The listing builds one solid part. Answer for the finished solid, in the listing's coordinates (mm). A direction names the side the tool comes from. Round coordinates to 2 decimals unless told otherwise and drop trailing zeros. Order: outer loops, then holes, each group sorted by start corner. A loop starts at its lowest first (then second) coordinate and runs counter-clockwise, first axis right, second up. Notation, with made-up numbers: (-25.75, 51) - (19.25, 51) arc R9 ccw to (19.25, 59) - close; hole circle Ø11 at (41.25, -33). An arc over 180 degrees is marked (long way). Use CSV: the item, a comma, the result in double quotes. Start each with the question number.
Item 1: Find section A-A, the plane x = 0. Give the vertices of the cut face in (y, z), plus the area to 3 significant figures.
Item 2: Find section B-B, the plane z = 0. Give the vertices of the cut face in (x, y).
Item 3: Find section C-C, the plane x = 14. Give the vertices of the cut face in (y, z).
Item 4: Determine the mould class of faces 1 (the cylindrical face through (-10.74, 15.19, -2.38)), 2 (the cylindrical face through (16.539, 6.134, 11.127)), 3 (the flat face through (-5, 7.3, -10)) for opening direction X: +X half, -X half, draft (parallel to the pull), parting line (faces both ways), or undercut.
Item 5: Straight lines are drawn through the part: line 1 along Y through (x, z) = (-6.5, 13.5); line 2 along Z through (x, y) = (-4, 13); line 3 along X through (y, z) = (13.75, 6.5). For each, find the intervals that lie inside material, in ascending order. Write a range as [from, to].
Item 6: Flat-ended cylindrical pins translate along their axes: P1, Ø6, axis at x = 14.71, z = 9.14, coming from the -Y side; P2, Ø1, axis at x = 17, z = 17, coming from the -Y side; P3, Ø5, axis at x = 8, z = 17.5, coming from the +Y side; P4, Ø2, axis at x = 6, y = 17, coming from the +Z side. Find the tip coordinate at first contact, or state that the pin passes through.
Item 7: For faces 4 (the cylindrical face through (-2.44, 11.49, 0.54)), 5 (the flat face through (-5, 5, -10)), determine the directions among +Z, -Z, +X, -X, +Y, -Y from which every point of the face is accessible in a straight line to the end or side of a thin tool.
Item 8: Find section D-D, the plane y = 21.25. Give the vertices of the cut face in (x, z), plus the area to 3 significant figures.
```python
from build123d import *

# Parameters (mm, degrees)
SKETCH1_R           = 11
BOSS_EXTRUDE1_DEPTH = 5
SKETCH2_R           = 22.25
BOSS_EXTRUDE2_DEPTH = 2.3
SKETCH3_R           = 11
BOSS_EXTRUDE3_DEPTH = 16
SKETCH4_R           = 2.5
CUT_EXTRUDE1_DEPTH  = 30
SKETCH5_R           = 2.7
CUT_EXTRUDE2_DEPTH  = 16


with BuildPart() as part:
    # Sketch1 → Boss-Extrude1 (new body)
    with BuildSketch(Plane(origin=(0, 0, 0), x_dir=(1, 0, 0), z_dir=(0, 1, 0))):
        with Locations(Location((0, 0, 0), (0, 0, 270))):
            Circle(SKETCH1_R)
    extrude(amount=BOSS_EXTRUDE1_DEPTH)

    # Sketch2 → Boss-Extrude2 (add)
    with BuildSketch(Plane(origin=(0, 5, 0), x_dir=(1, 0, 0), z_dir=(0, 1, 0))):
        with Locations(Location((0, 0, 0), (0, 0, 270))):
            Circle(SKETCH2_R)
    extrude(amount=BOSS_EXTRUDE2_DEPTH)

    # Sketch3 → Boss-Extrude3 (add)
    with BuildSketch(Plane(origin=(0, 7.3, 0), x_dir=(1, 0, 0), z_dir=(0, 1, 0))):
        with Locations(Location((0, 0, 0), (0, 0, 270))):
            Circle(SKETCH3_R)
    extrude(amount=BOSS_EXTRUDE3_DEPTH)

    # Sketch4 → Cut-Extrude1 (cut)
    with BuildSketch(Plane.XZ):
        with Locations(Location((0, 0, 0), (0, 0, 270))):
            Circle(SKETCH4_R)
    extrude(amount=-CUT_EXTRUDE1_DEPTH, mode=Mode.SUBTRACT)

    # Sketch5 → Cut-Extrude2 (cut)
    with BuildSketch(Plane.XZ.offset(-5)):
        with Locations(Location((-15.270211919, 8.174388537, 0), (0, 0, 270))):
            Circle(SKETCH5_R)
        with Locations(Location((14.714334093, 9.137197175, 0), (0, 0, 270))):
            Circle(SKETCH5_R)
        with Locations(Location((0.555877826, -17.311585711, 0), (0, 0, 270))):
            Circle(SKETCH5_R)
    extrude(amount=-CUT_EXTRUDE2_DEPTH, mode=Mode.SUBTRACT)


solid = part.part
```
Worked out:
1,outline,"(0, -11) - (5, -11) - (5, -14.67) - (7.3, -14.67) - (7.3, -11) - (23.3, -11) - (23.3, -2.5) - (0, -2.5) - close; (0, 2.5) - (23.3, 2.5) - (23.3, 11) - (7.3, 11) - (7.3, 22.25) - (5, 22.25) - (5, 11) - (0, 11) - close; (5, -22.25) - (7.3, -22.25) - (7.3, -19.95) - (5, -19.95) - close"
1,area,"436 mm²"
2,outline,"(-22.25, 5) - (-11, 5) - (-11, 0) - (-2.5, 0) - (-2.5, 23.3) - (-11, 23.3) - (-11, 7.3) - (-22.25, 7.3) - close; (2.5, 0) - (11, 0) - (11, 5) - (22.25, 5) - (22.25, 7.3) - (11, 7.3) - (11, 23.3) - (2.5, 23.3) - close"
3,outline,"(5, -17.29) - (7.3, -17.29) - (7.3, 6.53) - (5, 6.53) - close; (5, 11.74) - (7.3, 11.74) - (7.3, 17.29) - (5, 17.29) - close"
4,face 1,"parting line"
4,face 2,"undercut"
4,face 3,"draft"
5,line 1,"y = [5, 7.3]"
5,line 2,"z = [-10.25, 10.25]"
5,line 3,"x = [-8.87, 8.87]"
6,P1,"stops at y = 5"
6,P2,"passes through"
6,P3,"stops at y = 7.3"
6,P4,"stops at z = 9.8"
7,face 4,"+Y, -Y"
7,face 5,"-Y"
8,outline,"circle Ø22 at (0, 0); hole circle Ø5 at (0, 0)"
8,area,"360 mm²"
